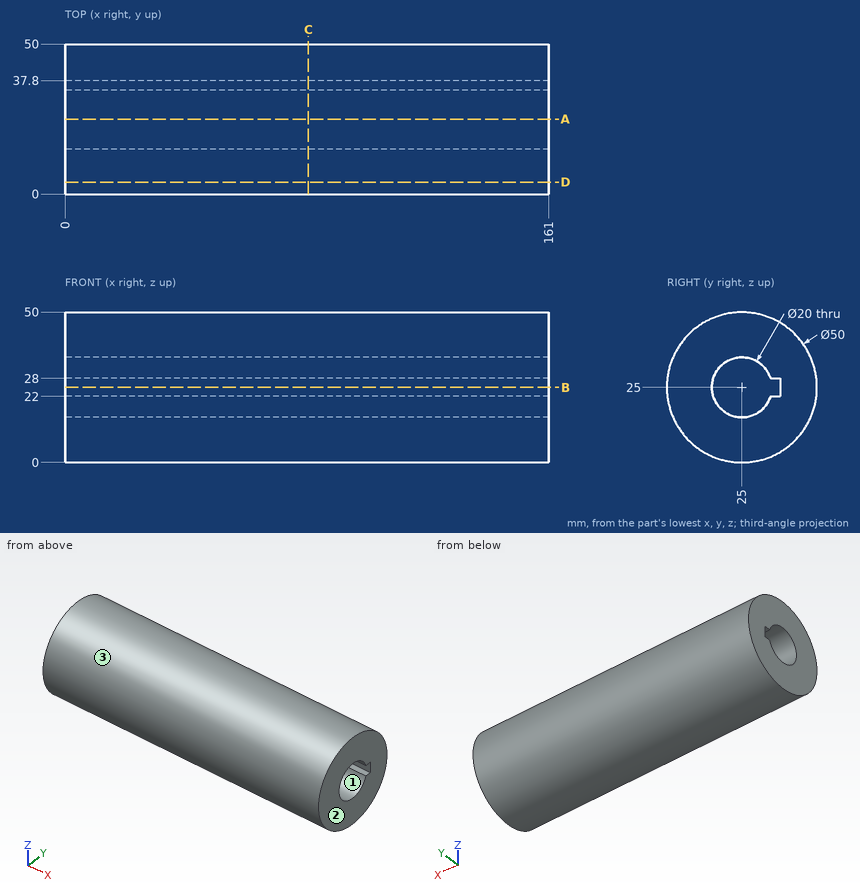
Design review of the part shown in the three views and the two pictorial views. Dimensions are in mm from the part's minimum x, y and z. Round coordinates to 2 decimals unless told otherwise and drop trailing zeros. Write each loop counter-clockwise with the first axis right and the second up, starting at its lowest first coordinate (ties: lowest second). Pieces come first, ordered by that corner, then holes. Notation, with made-up numbers: (11.25, 10.5) -> (21.25, 10.5) arc R26 cw to (21.25, 35.5) -> close; hole circle Ø11 at (89, 74). An arc over 180 degrees is marked (long way). Write item = value, one per line. Start each with the question number.
1) Take a section at A-A, the plane y = 25. State the section outline as (x, z) points.
2) Take a section at B-B, the plane z = 25. State the section outline as (x, y) points.
3) Clearance check with flat-ended pins moving along their axes: pin 1 (2 mm diameter, centred on x = 38.5, z = 21, fed in from +Y); pin 2 (5 mm diameter, centred on x = 30.5, z = 38.5, fed in from +Y); pin 3 (1 mm diameter, centred on x = 62.5, y = 36.5, fed in from +Z); pin 4 (8 mm diameter, centred on y = 37.5, z = 6.5, fed in from -X). State where each tip first meets the part, or that it passes through.
4) Take a section at C-C, the plane x = 81. State the section outline as (y, z) points.
5) Mouldability with a two-part tool opening along Y and no side actions: class the marked faces 1, 2 and 3 as +Y half, -Y half, draft (parallel to the pull), parting line (faces both ways), or undercut.
6) Wall thickness on probe 1 along Y at (x, z) = (54, 25); probe 2 along Y at (x, z) = (85, 21); probe 3 along Z at (x, y) = (93.5, 24): over which ranges is each line inside the solid? List them lowest first. Write a range as from..to.
7) Take a section at D-D, the plane y = 4. State the section outline as (x, z) points.
Results list:
q1.outline = (0, 0) -> (161, 0) -> (161, 15) -> (0, 15) -> close; (0, 35) -> (161, 35) -> (161, 50) -> (0, 50) -> close
q2.outline = (0, 0) -> (161, 0) -> (161, 15) -> (0, 15) -> close; (0, 37.8) -> (161, 37.8) -> (161, 50) -> (0, 50) -> close
q3.pin_1 = 49.82
q3.pin_2 = 47.45
q3.pin_3 = 47.45
q3.pin_4 = 0
q4.outline = circle Ø50 at (25, 25); hole (34.54, 22) -> (37.8, 22) -> (37.8, 28) -> (34.54, 28) arc R10 ccw (long way) to start
q5.face_1 = undercut
q5.face_2 = draft
q5.face_3 = parting line
q6.probe_1 = 0..15, 37.8..50
q6.probe_2 = 0.32..15.83, 34.17..49.68
q6.probe_3 = 0.02..15.05, 34.95..49.98
q7.outline = (0, 11.44) -> (161, 11.44) -> (161, 38.56) -> (0, 38.56) -> close
